```python
from build123d import *

# Parameters (mm, degrees)
BOSS_EXTRUDE2_DEPTH = 3
SKETCH2_W           = 8.689494808
SKETCH2_H           = 5.818516347
CUT_EXTRUDE1_DEPTH  = 3


with BuildPart() as part:
    # Model → Boss-Extrude2 (new body)
    with BuildSketch(Plane.XY):
        Polygon((0, 0), (30, 0), (30, 80), (40, 80), (15, 105), (-10, 80), (0, 80), align=None)
    extrude(amount=BOSS_EXTRUDE2_DEPTH)

    # Sketch2 → Cut-Extrude1 (cut)
    with BuildSketch(Plane.XY.offset(3)):
        with Locations((15.580557609, 86.224591519)):
            Rectangle(SKETCH2_W, SKETCH2_H)
    extrude(amount=-CUT_EXTRUDE1_DEPTH, mode=Mode.SUBTRACT)


solid = part.part
```
Geometry check sheet. Reference: the model listing, model coordinates, mm. A direction names the side the tool comes from. Coordinates: 2 decimals unless noted, no trailing zeros. Order: outer loops, then holes, each group sorted by start corner. A loop starts at its lowest first (then second) coordinate and runs counter-clockwise, first axis right, second up. Notation, with made-up numbers: M -27.5,70.5 L 22.5,70.5 A14 cw 22.5,84.5 Z; hole C 27.5,42.25 d9. An arc over 180 degrees is marked long. One line per question, with ' | ' between items. Start each with the question number.
Item 1: Gauge pin test, flat ends, axial feed: pin 1 (1.5 mm diameter, centred on x = -6, z = 2, fed in from -Y); pin 2 (1 mm diameter, centred on x = -3, z = 1.5, fed in from +Y); pin 3 (1.5 mm diameter, centred on y = 53.5, z = 2, fed in from +X). Record the tip position at first contact, or that the pin passes through.
Item 2: Material ranges on L1, parallel to X at y = 62, z = 0.45; L2, parallel to Y at x = -1, z = 0.45; L3, parallel to Y at x = 1, z = 1.6, recorded low to high. Write a range as [from, to].
Item 3: Set-up check for faces 1 (the flat face through (11.236, 86, 2)), 2 (the flat face through (3, 93, 1)), 3 (the flat face through (-5, 80, 1)), 4 (the flat face through (35, 80, 1)): record each of +Z, -Z, +X, -X, +Y, -Y from which the full face is reachable in a straight line by a thin tool's end or side.
Item 4: Cross-section at A-A on x = 13. Enter the section's corners in (y, z), then the cut area to 3 significant figures.
Item 5: Draft check along Y on faces 5 (the flat face through (30, 39, 1)), 6 (the flat face through (28, 92, 1)), 7 (the flat face through (16, 83.315, 2)). Enter one of: pulls with the +Y half, pulls with the -Y half, needs draft (parallel to the pull), parting line crosses it, or undercut.
Item 6: Cross-section at C-C on y = 15. Enter the section's corners in (x, z), then the cut area to 3 significant figures.
Item 7: Cross-section at B-B on x = 32. Enter the section's corners in (y, z).
Findings:
1) pin 1: stops at y = 80 | pin 2: stops at y = 87.5 | pin 3: stops at x = 30
2) L1: x = [0, 30] | L2: y = [80, 89] | L3: y = [0, 91]
3) face 1: +Z, -Z | face 2: +Z, -Z, -X, +Y | face 3: +Z, -Z, -X, -Y | face 4: +Z, -Z, +X, -Y
4) outline: M 0,0 L 83.32,0 L 83.32,3 L 0,3 Z; M 89.13,0 L 103,0 L 103,3 L 89.13,3 Z | area: 292 mm²
5) face 5: needs draft | face 6: pulls with the +Y half | face 7: undercut
6) outline: M 0,0 L 30,0 L 30,3 L 0,3 Z | area: 90.0 mm²
7) outline: M 80,0 L 88,0 L 88,3 L 80,3 Z
